Solid Edge part; units mm, degrees
sketch "Sketch1" plane through (0, 0, 0) normal (0, -1, 0) x (1, 0, 0)
  line L0 (2.75, 3) -> (2.75, 0)
  line L1 (2.75, 0) -> (1.8, 0)
  line L2 (1.8, 0) -> (1.5, -0.5196)
  line L3 (1.5, -0.5196) -> (1.5, -6)
  line L4 (1.5, -6) -> (0, -6)
  line L5 (1.25, 1.7) -> (0, 0.9783)
  line L6 (1.25, 3) -> (1.25, 1.7)
  line L7 (2.75, 3) -> (1.25, 3)
revolve "RevolvedProtrusion1" add sketch "Sketch1" angle 360 about axis through (0, 0, -6) along (0, 0, 1)
cosmetic_thread "Thread1"
chamfer "Chamfer_1" distance 0.25 angle 45 1 edges at (-1.5, 0, -6)
fillet "Round_1" radius 0.3 2 edges at (-2.75, 0, 0) (-2.75, 0, 3)
sketch "Sketch2" plane through (0, 0, 3) normal (0, 0, 1) x (0, 1, 0)
  line L0 (-1.25, 0.7217) -> (-1.25, -0.7217)
  line L1 (0, -1.4434) -> (-1.25, -0.7217)
  line L2 (1.25, -0.7217) -> (0, -1.4434)
  line L3 (1.25, 0.7217) -> (1.25, -0.7217)
  line L4 (0, 1.4434) -> (1.25, 0.7217)
  line L5 (-1.25, 0.7217) -> (0, 1.4434)
extrude "Cutout1" cut sketch "Sketch2" against normal up to vertex (1.3 mm away)
properties material "Galvanized steel"
Verification items for the finished model (mm, model axes). A direction names the side the tool comes from. Coordinates: 2 decimals unless noted, no trailing zeros. Write each loop counter-clockwise with the first axis right and the second up, starting at its lowest first coordinate (ties: lowest second). Pieces come first, ordered by that corner, then holes. Notation, with made-up numbers: M 68.25,28 L 79.25,28 A16 ccw 79.25,36 Z; hole C 10.5,52.5 d10. An arc over 180 degrees is marked long. Answer as a JSON object with one key per item and string values. Group by question number.
(1) Release check for a two-part mould opening along X. For faces 4 (the face through (1.08, 0.63, 2.36)), 5 (the face through (-0.596, 2.685, 1.483)), 6 (the face through (0, 2, 0)) record: +X half, -X half, draft (parallel to the pull), parting line (faces both ways), or undercut.
(2) Cross-section at B-B, the plane z = 1.5. Record the cut outline in (x, y).
(3) Material ranges on line 1 (Z direction, x = -2.3, y = 0.6); line 2 (X direction, y = 0.25, z = 1.25); line 3 (Y direction, x = -0.05, z = -4.5), recorded low to high.
(4) Gauge pin test, flat ends, axial feed: pin 1 (1.5 mm diameter, centred on y = 2, z = -3.5, fed in from +X); pin 2 (1.5 mm diameter, centred on y = 1, z = -2, fed in from -X); pin 3 (0.7 mm diameter, centred on x = 0.5, y = -0.5, fed in from +Z). Record the tip position at first contact, or that the pin passes through.
(5) Tool access check on faces 1 (the face through (1.1, -1.1, 3)), 2 (the face through (-1.5, -0.07, -3.17)), 3 (the face through (-1.088, 0.616, 2.359)). Record the directions out of +Z, -Z, +X, -X, +Y, -Y that give a thin tool (end or side, any length) a straight path to the whole face; none if there is none.
(6) Cross-section at A-A, the plane z = -5. Record the cut outline in (x, y), and give its area (3 significant figures).
Reply:
{
 "1": {"face 4": "undercut", "face 5": "parting line", "face 6": "draft"},
 "2": {"outline": "C 0,0 d5.5; hole C 0,0 d1.81"},
 "3": {"line 1": "0 to 3", "line 2": "-2.74 to -0.4, 0.4 to 2.74", "line 3": "-1.5 to 1.5"},
 "4": {"pin 1": "x = 0.83", "pin 2": "x = -1.48", "pin 3": "z = 1.59"},
 "5": {"face 1": "+Z, +X, -X, +Y, -Y", "face 2": "-Z", "face 3": "+Z"},
 "6": {"outline": "C 0,0 d3", "area": "7.07 mm²"}
}
